The listing builds one solid part. Answer for the finished solid, in the listing's coordinates (mm). A direction names the side the tool comes from. Round coordinates to 2 decimals unless told otherwise and drop trailing zeros. Order: outer loops, then holes, each group sorted by start corner. A loop starts at its lowest first (then second) coordinate and runs counter-clockwise, first axis right, second up. Notation, with made-up numbers: (23, -4) -> (71, -4) arc R8 cw to (71, 8) -> close; hole circle Ø7 at (-37, 44.25). An arc over 180 degrees is marked (long way). Return JSON: item names as keys, results as strings. Group by question number.
(1) Determine the mould class of faces 1 (the face through (-6.965, 2.944, -0.053)), 2 (the face through (-2.54, 138.02, 0.95)), 3 (the face through (-4.5, -3.2, -0.2)) for opening direction Z: +Z half, -Z half, draft (parallel to the pull), parting line (faces both ways), or undercut.
(2) The part is cut by section B-B (x = 0). Determine the outline of the cut face in (y, z).
(3) Consider line 1 (X direction, y = 135.5, z = 2); line 2 (Y direction, x = -3.5, z = 2); line 3 (Y direction, x = -2.75, z = -0.5). Determine where each line is inside the solid, lowest interval first. Write a range as [from, to].
(4) Which of the six approach directions +Z, -Z, +X, -X, +Y, -Y give full straight-line access (tool end or side, diameter ignored) to faces 4 (the face through (-4, 72, 2)), 5 (the face through (0, 132.85, 2)), 6 (the face through (0, 75, -2)), 7 (the face through (-3, -2, 5.5))?
(5) Each of these flat-tipped pins is pushed along its axis until it touches: pin 1 (8 mm diameter, centred on x = 0.5, y = 113.5, fed in from -Z); pin 2 (5 mm diameter, centred on x = -6.5, z = -1, fed in from -Y); pin 3 (1.8 mm diameter, centred on y = 73, z = 3.5, fed in from -X). Where does it stop, or does it pass through?
(6) The part is cut by section A-A (y = 63.5). Determine the outline of the cut face in (x, z).
(7) The part is cut by section C-C (x = -6.5). Determine the outline of the cut face in (y, z), plus the area to 3 significant figures.
Autodesk Inventor part; units mm, degrees
ref_plane "Plano de trabajo2" through (0, 177.05, 0) normal (0, 1, 0) x (-1, 0, 0)
ref_plane "YZ Plane" through (0, 0, 0) normal (1, 0, 0) x (0, 1, 0)
ref_plane "XY Plane" through (0, 0, 0) normal (0, 0, 1) x (1, 0, 0)
sketch "Boceto1" plane through (0, 0, 0) normal (1, 0, 0) x (0, 1, 0)
  circle A0 centre (0, 0) radius 5
  line L0 (0, 0) -> (0, 6)
  line L1 (0, 6) -> (-4, 6)
  line L2 (-5, 5) -> (-5, 0)
  line L3 (0, 6) -> (181.05, 6)
  line L4 (181.05, 6) -> (187.5, 6)
  line L5 (187.5, 6) -> (189.65, 6)
  line L6 (190.65, 5) -> (190.65, -1)
  line L7 (189.65, -2) -> (4.5826, -2)
  arc A1 (-4, 6) -> (-5, 5) centre (-4, 5) ccw
  arc A2 (190.65, 5) -> (189.65, 6) centre (189.65, 5) ccw
  arc A3 (189.65, -2) -> (190.65, -1) centre (189.65, -1) ccw
  line L8 (3.5707, -3.5) -> (-3.5707, -3.5)
  point P0 (-5, 6)
  point P1 (190.65, 6)
  point P2 (190.65, -2)
  dimension "d0" = 10
  dimension "d1" = 6
  dimension "d2" = 5
  dimension "d3" = 181.05
  dimension "d4" = 6.45
  dimension "d5" = 3.15
  dimension "d6" = 8
  dimension "d7" = 1
  dimension "d8" = 1
  dimension "d45" = 1.5
extrude "Extrusión1" add sketch "Boceto1" along normal mid plane 8 contours A0 L8 | L2 A1 L1 L0 A0 | L0 L3 L4 L5 A2 L6 A3 L7 A0 picked at (0, -0.6667)
fillet "Empalme1" radius 1 18 edges at (-4, 190.3571, 5.7071) (-4, 190.65, 2) (-4, 190.3571, -1.7071) (-4, 97.1163, -2) (-4, -4.7071, 5.7071) (-4, -5, 2.5) (-4, -4.6289, -1.8903) (-4, 4.1451, -2.7962) (-4, 92.825, 6) (4, -4.7071, 5.7071) (4, -5, 2.5) (4, -4.6289, -1.8903) (4, 4.1451, -2.7962) (4, 190.3571, 5.7071) (4, 190.65, 2) (4, 190.3571, -1.7071) (4, 97.1163, -2) (4, 92.825, 6)
sketch "Boceto2" plane through (-4, 0, 0) normal (-1, 0, 0) x (0, 0, 1)
  circle A0 centre (0, 0) radius 5.5
  line L0 (4.7631, 2.75) -> (-2, 14.4641)
  line L1 (-2, 189.65) -> (-2, 4.5826)
  line L2 (5.5, 0) -> (5.5, -5.5)
  line L3 (0, -5) -> (5, -5)
  line L4 (0, -5.5) -> (5.5, -5.5)
  line L5 (-2, 14.4641) -> (-2, 5.1235)
  dimension "d12" = 11
  dimension "d13" = 30
extrude "Extrusión2" cut sketch "Boceto2" against normal blind 2.5
sketch "Boceto3" plane through (0, 0, 0) normal (0, 0, 1) x (1, 0, 0)
  line L0 (-3, 190.65) -> (3, 190.65)
  line L1 (0, 190.65) -> (0, 181.05)
  line L2 (1.4, 190.65) -> (1.4, 181.05)
  line L3 (-1.4, 190.65) -> (-1.4, 181.05)
  line L4 (1.4, 190.65) -> (-1.4, 190.65)
  line L5 (0, 181.05) -> (1.4, 181.05)
  line L6 (0, 181.05) -> (-1.4, 181.05)
  point P0 (0, 0)
  dimension "d16" = 9.6
  dimension "d17" = 1.4
  dimension "d18" = 1.4
extrude "Extrusión3" cut sketch "Boceto3" along normal mid plane 16
fillet "Empalme4" radius 1 2 edges at (-1.4, 181.05, 2) (1.4, 181.05, 2)
sketch "Boceto11" plane through (0, 0, 0) normal (1, 0, 0) x (0, 1, 0)
  line L0 (0, 0) -> (0, 6)
  line L1 (0, 6) -> (181.05, 6)
  line L2 (189.65, 6) -> (-4, 6)
  line L3 (181.05, 6) -> (187.5, 6)
  line L4 (187.5, 6) -> (187.5, 0.55)
  circle A0 centre (187.5, 0.55) radius 1.15
  dimension "d66" = 6
  dimension "d67" = 181.05
  dimension "d68" = 6.45
  dimension "d69" = 5.45
  dimension "d70" = 2.3
extrude "Extrusión9" cut sketch "Boceto11" along normal through all both and the other way through all
sketch "Boceto6" plane through (0, 0, 0) normal (0, 0, 1) x (1, 0, 0)
  line L0 (0, 0) -> (-1.5, 0)
  line L1 (-1.5, 0) -> (-1.5, -3)
  line L2 (-1.5, -5) -> (-1.5, 4.5826)
  line L3 (-1.5, -3) -> (-4.5, -3)
  line L4 (-1.5, 0) -> (-9.5, 0)
  line L5 (-4.5, -3) -> (-4.5, -3.5)
  line L6 (-9.5, 0) -> (-9.5, -2.3732)
  line L7 (-9.5, -2.3732) -> (-4.5, -3.5)
  dimension "d27" = 1.5
  dimension "d28" = 3
  dimension "d29" = 3
  dimension "d30" = 8
  dimension "d31" = 0.5
  dimension "d32" = 2.3732
revolve "Revolución1" add sketch "Boceto6" angle 360 about axis through (-1.5, 0, 0) along (-1, 0, 0)
sketch "Boceto7" plane through (0, 0, 0) normal (0, 0, 1) x (1, 0, 0)
  line L0 (0, 0) -> (-1.5, 0)
  line L1 (-1.5, 0) -> (-4.5, 0)
  line L2 (-4.5, 0) -> (-9.5, 0)
  line L3 (-9.5, 0) -> (-9.5, -1)
  line L4 (-9.5, 2.3732) -> (-9.5, -2.3732)
  line L5 (-9.5, -1) -> (-2.5, -1)
  line L6 (-2.5, -1) -> (-2.5, 1)
  line L7 (-2.5, 1) -> (-9.5, 1)
  line L8 (-9.5, 1) -> (-9.5, 0)
  point P0 (-9.5, 1)
  dimension "d34" = 1.5
  dimension "d35" = 3
  dimension "d36" = 5
  dimension "d37" = 1
  dimension "d38" = 7
  dimension "d39" = 2
extrude "Extrusión5" cut sketch "Boceto7" along normal mid plane 7
fillet "Empalme2" radius 1 2 edges at (-2.5, -1, 0) (-2.5, 1, 0)
ref_plane "Plano de trabajo2" through (0, 177.05, 0) normal (0, 1, 0) x (-1, 0, 0)
sketch "Boceto8" plane through (0, 177.05, 0) normal (0, 1, 0) x (-1, 0, 0)
  line L0 (0, 0) -> (0, 2)
  line L1 (16, 18) -> (-16, 18)
  line L2 (-16, 18) -> (-16, -14)
  line L3 (-16, -14) -> (16, -14)
  line L4 (16, -14) -> (16, 18)
  line L5 (16, 18) -> (-16, -14) construction
  line L6 (-16, 18) -> (16, -14) construction
  point P0 (0, 0)
  dimension "d49" = 2
  dimension "d50" = 32
  dimension "d51" = 32
  dimension "d78" = 0
extrude "Extrusión6" cut sketch "Boceto8" against normal blind 34
sketch "Boceto9" plane through (0, 177.05, 0) normal (0, -1, 0) x (-1, 0, 0)
  line L0 (3, -6) -> (-3, -6)
  line L1 (0, 0) -> (0, -2)
  circle A0 centre (0, -2) radius 2.75
  point P0 (0, 0)
  point P1 (-2.6, -6)
  dimension "d55" = 2
  dimension "d56" = 5.5
  dimension "d79" = 0
  dimension "d80" = 0
extrude "Extrusión7" cut sketch "Boceto9" along normal blind 44.2
sketch "Boceto10" plane through (0, 177.05, 0) normal (0, -1, 0) x (-1, 0, 0)
  circle A0 centre (0, -2) radius 2.6
  circle A1 centre (0, -2) radius 3
  point P0 (0, 0)
  dimension "d59" = 6
extrude "Extrusión8" [suppressed]
fillet "Empalme3" [suppressed]
sketch "Boceto13" plane through (0, 143.05, 0) normal (0, 1, 0) x (1, 0, 0)
  line L0 (16, -16) -> (-16, -16)
  line L1 (-16, -16) -> (-16, 16)
  line L2 (-16, 16) -> (16, 16)
  line L3 (16, 16) -> (16, -16)
  line L4 (16, -16) -> (-16, 16) construction
  line L5 (-16, -16) -> (16, 16) construction
  point P0 (0, 0)
  dimension "d81" = 32
  dimension "d82" = 32
extrude "Extrusión10" cut sketch "Boceto13" along normal blind 181.05
sketch "Boceto14" plane through (0, 0, 0) normal (1, 0, 0) x (0, 1, 0)
  line L0 (0, 0) -> (0, 6)
  line L1 (0, 6) -> (137.85, 6)
  line L2 (137.85, 6) -> (137.85, 2)
  circle A0 centre (137.85, 2) radius 0.5
  dimension "d85" = 6
  dimension "d86" = 137.85
  dimension "d87" = 4
  dimension "d88" = 1
extrude "Extrusión11" cut sketch "Boceto14" along normal through all both and the other way through all
equation "\"d0\" = width_r3"
equation "\"d1\" = 0.5 * width_r3 + offset"
equation "\"d3\" = lenght_body_link - 0.5 * width_r3"
equation "\"d4\" = shaft_y"
equation "\"d45\" = 1.5 * offset"
equation "\"d9\" = width_link"
equation "\"d12\" = width_r3 + offset"
equation "\"d14\" = 0.5 * width_link - 0.5 * t_thikness"
equation "\"d16\" = 0.5 * Djoint_shaft + 2 * offset + shaft_y"
equation "\"d17\" = 0.25 * offset + 0.5 * wire_D"
equation "\"d18\" = 0.25 * offset + 0.5 * wire_D"
equation "\"d19\" = 2 * width_link"
equation "\"d63\" = offset"
equation "\"d27\" = 0.5 * t_thikness"
equation "\"d28\" = 0.5 * sj_diam_shaft"
equation "\"d29\" = t_thikness"
equation "\"d30\" = t_thikness + sj_head_height"
equation "\"d31\" = 0.5 * sj_head_D - 0.5 * sj_diam_shaft"
equation "\"d32\" = 0.5 * sj_head_d"
equation "\"d34\" = 0.5 * t_thikness"
equation "\"d35\" = t_thikness"
equation "\"d36\" = sj_head_height"
equation "\"d37\" = 0.5 * sj_groove"
equation "\"d38\" = sj_groove_deep"
equation "\"d39\" = sj_groove"
equation "\"d40\" = sj_head_D"
equation "\"d46\" = 0.5 * sj_groove"
equation "\"d52\" = spring_lenght + 3 * thikness"
equation "\"d59\" = spring_int_d"
equation "\"d60\" = thikness"
equation "\"d62\" = offset"
equation "\"offset\" = 1"
equation "\"wire_D\" = 2.3"
equation "\"width_link\" = 8"
equation "\"Djoint_shaft\" = 2.3"
equation "\"shaft_x\" = 1.45"
equation "\"shaft_y\" = 6.45"
equation "\"lenght_body_link\" = 186.05"
equation "\"m2_theta3f\" = -60deg"
equation "\"width_r3\" = 10"
equation "\"t_thikness\" = 3"
equation "\"sj_diam_shaft\" = 6"
equation "\"sj_groove\" = 2"
equation "\"sj_groove_deep\" = 7"
equation "\"sj_head_D\" = 7"
equation "\"sj_head_d\" = 4.7464"
equation "\"sj_head_height\" = 5"
equation "\"thikness\" = 2"
equation "\"spring_int_d\" = 6"
equation "\"spring_lenght\" = 28"
equation "\"r1\" = 5.55"
equation "\"r2o\" = 59.75"
equation "\"delta_y\" = 6"
equation "\"wire_d\" = 1"
equation "\"width_ang_spring\" = 5"
equation "\"spring_int_diam\" = 8.5"
equation "\"spring_ext_diam\" = 10.5"
equation "\"r3\" = 8.25"
equation "\"r3R\" = 4.75"
equation "\"r3T\" = 6.74537"
equation "\"alpha\" = 54.847297deg"
equation "\"alpha2\" = 270deg"
equation "\"theta3_recogido\" = 305.152703deg"
equation "\"delta_theta_3\" = 45deg"
equation "\"joint_width\" = 12"
equation "\"joint_radius\" = 7.75"
equation "\"shaft_width\" = 15"
equation "\"shaft_joint_diameter\" = 7.75"
equation "\"separation_space\" = 0.5"
equation "\"height_finger\" = 42"
equation "\"cell_screw_head_diameter\" = 4"
equation "\"cell_screw_diameter\" = 2"
equation "\"cell_space\" = 2"
equation "\"cell_width\" = 6"
equation "\"cell_theta_position\" = 60deg"
equation "\"cell_thikness\" = 1"
equation "\"cell_lenght\" = 37"
equation "\"cell_z_space\" = 5"
equation "\"Dt\" = 1.05949"
equation "\"lenght_bar_support\" = 201.65"
equation "\"wire_spring_d\" = 1"
equation "\"trigger_offset\" = 2"
equation "\"m2_theta2o\" = 107deg"
equation "\"m2_r2\" = 28"
equation "\"e\" = 9"
equation "\"So\" = 17"
equation "\"m2_theta3o\" = -30deg"
equation "\"m2_r3\" = 19.75"
equation "\"m2_delta_theta1\" = 15deg"
equation "\"trigger_thumb_lenght\" = 6"
equation "\"width_r12\" = 8"
equation "\"m2_r1\" = 25.2"
equation "\"r3_thikness\" = 3.5"
equation "\"tg_width\" = 4"
equation "\"pivot_screw_d\" = 4"
equation "\"pivot_diameter\" = 7"
equation "\"sf_lenght\" = 9.5"
equation "\"sf_base\" = 3"
equation "\"sf_head_height\" = 3"
equation "\"sf_head_width\" = 4.5"
equation "\"sf_head_offset\" = 0.25"
equation "\"sf_head_grip_width\" = 2"
equation "\"sf_head_angle\" = 45deg"
equation "\"sf_thikness\" = 5"
equation "\"screw_Dhead\" = 8"
equation "\"screw_d\" = 4"
equation "\"screw_lenght\" = 12"
equation "\"screwJ_base_D\" = 9"
equation "\"screwJ_top_D\" = 13"
equation "\"gj_D\" = 6"
equation "\"gj_d\" = 4"
equation "\"gj_out_section\" = 6"
equation "\"agarradera_theta\" = 60deg"
equation "\"agarradera_width\" = 4"
equation "\"sfbox_theta1\" = 60deg"
equation "\"sfbox_theta2\" = 45deg"
equation "\"position\" = 39.13077"
equation "\"fat_width_slider\" = 2"
equation "\"sfbox_tip_width\" = 2.5"
equation "\"flex_separation_theta\" = 60deg"
equation "\"sf_flex_separation\" = 38.66667"
equation "\"ext_width_slider\" = 3.5"
equation "\"sf_box_width\" = 1.5"
equation "\"slim_width_slider\" = 1.5"
equation "\"sfbox_width\" = 1.5"
equation "\"int_width_slider\" = 2"
equation "\"box_fat_slider_lenght\" = 67"
equation "\"box_slim_slider_lenght\" = 116"
equation "\"thikness_box\" = 1.5"
equation "\"box_in_height\" = 35"
equation "\"box_in_width\" = 72"
equation "\"box_in_deep\" = 77"
equation "\"agarradera_position\" = 82.13077"
properties part number "Eslabón conector M2" material "Plástico PPS"
Answer below:
{
 "1": {"face 1": "parting line", "face 2": "undercut", "face 3": "draft"},
 "2": {"outline": "(-5, 0) arc R5 ccw to (-3.57, -3.5) -> (3.57, -3.5) arc R5 ccw to (4.58, -2) -> (143.05, -2) -> (143.05, -0.75) -> (132.85, -0.75) -> (132.85, 4.75) -> (143.05, 4.75) -> (143.05, 6) -> (-4, 6) arc R1 ccw to (-5, 5) -> close"},
 "3": {"line 1": "x = [-4, -2.75], [2.75, 4]", "line 2": "y = [-2.24, -1], [1, 2.24], [7.54, 137.35], [138.35, 143.05]", "line 3": "y = [-2.96, -0.66], [0.66, 2.96], [11.87, 143.05]"},
 "4": {"face 4": "+Z, -Z, -X, +Y", "face 5": "+Y", "face 6": "-Z, +X, -X, +Y", "face 7": "-X, -Y"},
 "5": {"pin 1": "stops at z = -2", "pin 2": "stops at y = -3.5", "pin 3": "stops at x = -4"},
 "6": {"outline": "(-4, -1) arc R1 ccw to (-3, -2) -> (3, -2) arc R1 ccw to (4, -1) -> (4, 5) arc R1 ccw to (3, 6) -> (-3, 6) arc R1 ccw to (-4, 5) -> close"},
 "7": {"outline": "(-1, -2.88) -> (-1, 2.88) arc R3.05 ccw to start; (1, -2.88) arc R3.05 ccw to (1, 2.88) -> close", "area": "17.2 mm²"}
}
